```python
from build123d import *

# Parameters (mm, degrees)
F0_W        = 62.0055571198
F0_H        = 91.1606
F2_W        = 43.9132880419
F2_H        = 91.28
F4_R        = 20
F5_R        = 20
F6_T1_DEPTH = 247.1570875446
F8_R        = 17.2017157063
F8_R_2      = 16.2487468326
F9_DEPTH    = 5
F10_DEPTH   = 5


# Not quite as in the source:
# - a fillet or chamfer that OpenCascade refuses, or shapes differently, is made with other operations: its cross-section is extruded or revolved along the edge and cut away or added


with BuildPart() as f3:
    # F0 (on Top) → F3 section 0
    with BuildSketch(Plane.XY):
        with Locations((3.4252367914, -5.9738955829)):
            Rectangle(F0_W, F0_H)
    # F2 (on offset) → F3 section 1
    with BuildSketch(Plane.XY.offset(20)):
        with Locations((12.6207480207, -6.1396389759)):
            Rectangle(F2_W, F2_H)
    loft()

    # F4
    f4_edges = [f3.edges().sort_by_distance(p)[0] for p in [
        (-9.335896, -6.139639, 20),
    ]]
    fillet(f4_edges, radius=F4_R)

    # F5
    f5_edges = [f3.edges().sort_by_distance(p)[0] for p in [
        (34.428015, -5.973896, 0),
    ]]
    fillet(f5_edges, radius=F5_R)

    # F6: fillet of radius 20 on 1 edges, made by hand

    # F6_s2 → F6_t1 (cut)
    with BuildSketch(Plane.XZ.offset(-117.6046481894)):
        with BuildLine():
            ThreePointArc((3.6217557404, 0), (-7.9875678865, 3.7143128813), (-15.2848254843, 13.4776395073))
            Line((-15.2848254843, 13.4776395073), (-27.5775417686, 0))
            Line((-27.5775417686, 0), (3.6217557404, 0))
        make_face()
    extrude(amount=F6_T1_DEPTH, mode=Mode.SUBTRACT)

    # F8 (on offset) → F9 (join)
    with BuildSketch(Plane.XY.offset(20)):
        with Locations((16.8321914971, -3.0107519124)):
            Circle(F8_R)
        with Locations((16.8321914971, -3.0107519124)):
            Circle(F8_R_2, mode=Mode.SUBTRACT)
        Polygon((5.5154971778, 6.8484889343), (5.5154971778, -13.2129238918), (10.5462484062, -3.106220687), align=None)
        Polygon((27.3772925138, -12.8699932247), (27.3772925138, 6.9342213683), (22.7957628667, -2.8306879103), align=None)
    extrude(amount=F9_DEPTH)

    # F8 (on offset) → F10 (join)
    with BuildSketch(Plane.XY.offset(20)):
        Polygon((17.0036572963, 9.8491283134), (10.6022227556, -3.106220687), (16.8321914971, -15.5277010053), (22.6763673127, -2.8306879103), align=None)
    extrude(amount=F10_DEPTH)


solid = f3.part
```
The listing builds one solid part. Answer for the finished solid, in the listing's coordinates (mm). A direction names the side the tool comes from. Give positions to 0.01 mm unless a question says otherwise; leave off trailing zeros. Loops run counter-clockwise (first coordinate to the right, second up) from the corner with the lowest first, then second, coordinate; pieces in that order, holes last. Notation, with made-up numbers: (10.25, 9) - (20.25, 9) arc R19 cw to (20.25, 30) - close; hole circle Ø2 at (2, 72.5). An arc over 180 degrees is marked (long way). Answer as CSV lines item,"result". Start each with the question number.
Item 1: The mould has two halves that part along Y. Classify faces 3 (the face through (33.24, 2.16, 22.46)), 4 (the face through (26, -18, 20)), 5 (the face through (13.848, 3.462, 22.465)): +Y half, -Y half, draft (parallel to the pull), parting line (faces both ways), or undercut.
Item 2: Each of these flat-tipped pins is pushed along its axis until it touches: pin 1 (12 mm diameter, centred on x = -5, y = -25.5, fed in from -Z); pin 2 (4 mm diameter, centred on y = 30.5, z = 16, fed in from +X); pin 3 (4 mm diameter, centred on y = -2.5, z = 23.5, fed in from -X). Where does it stop, or does it pass through?
Item 3: A cutting plane is placed at A-A on z = 22.75. Determine the outline of the cut face in (x, y).
Item 4: Find the intervals of material crossed by line 1 (X direction, y = 8, z = 21.5); line 2 (Y direction, x = 7.5, z = 19); line 3 (Y direction, x = 14.5, z = 12.75), in increasing order. Write a range as from..to.
Item 5: For faces 1 (the face through (9, -6, 0)), 2 (the face through (13.674, -9.23, 22.465)), determine the directions among +Z, -Z, +X, -X, +Y, -Y from which every point of the face is accessible in a straight line to the end or side of a thin tool.
Found:
1,face 3,"parting line"
1,face 4,"draft"
1,face 5,"undercut"
2,pin 1,"stops at z = 0.17"
2,pin 2,"stops at x = 34.48"
2,pin 3,"stops at x = -0.37"
3,outline,"circle Ø34.4 at (16.83, -3.01); (5.52, -13.21) - (10.55, -3.11) - (5.52, 6.85) - close; (10.6, -3.11) - (16.83, -15.53) - (22.68, -2.83) - (17, 9.85) - close; (22.8, -2.83) - (27.38, -12.87) - (27.38, 6.93) - close; hole circle Ø32.5 at (16.83, -3.01)"
4,line 1,"x = 3.62..4.88, 16.09..17.83, 28.78..30.05"
4,line 2,"y = -51.77..39.51"
4,line 3,"y = -51.7..39.54"
5,face 1,"-Z, +X, -X, +Y, -Y"
5,face 2,"+Z"
